Job drawing, mm, ordinate dimensions from the low corner. One solid piece. Give positions to 0.01 mm unless a question says otherwise; leave off trailing zeros. Loops run counter-clockwise (first coordinate to the right, second up) from the corner with the lowest first, then second, coordinate; pieces in that order, holes last. Notation, with made-up numbers: (5, 29.5) -> (40, 29.5) arc R20 cw to (40, 62.5) -> close; hole circle Ø7 at (11, 17). An arc over 180 degrees is marked (long way). Answer as a JSON object with one key per item and string values. Group by question number.
Q1. Drop a flat-ended pin along its axis: pin 1 (1.5 mm diameter, centred on x = 28.5, z = 57, fed in from -Y). Give the stop position or say it passes through.
Q2. Band-saw the part on C-C, the plane y = 0.2. Write the cut outline in (x, z).
Q3. Wall check: probe 1 along X at (y, z) = (0.2, 35); probe 2 along Z at (x, y) = (64, 0.35). Give the ranges that are in metal, low to high. Write a range as from..to.
Q4. Band-saw the part on A-A, the plane z = 35. Write the cut outline in (x, y).
Q5. Band-saw the part on B-B, the plane z = 7.5. Write the cut outline in (x, y).
Q6. Band-saw the part on D-D, the plane x = 7.5. Write the cut outline in (y, z), plus the area to 3 significant figures.
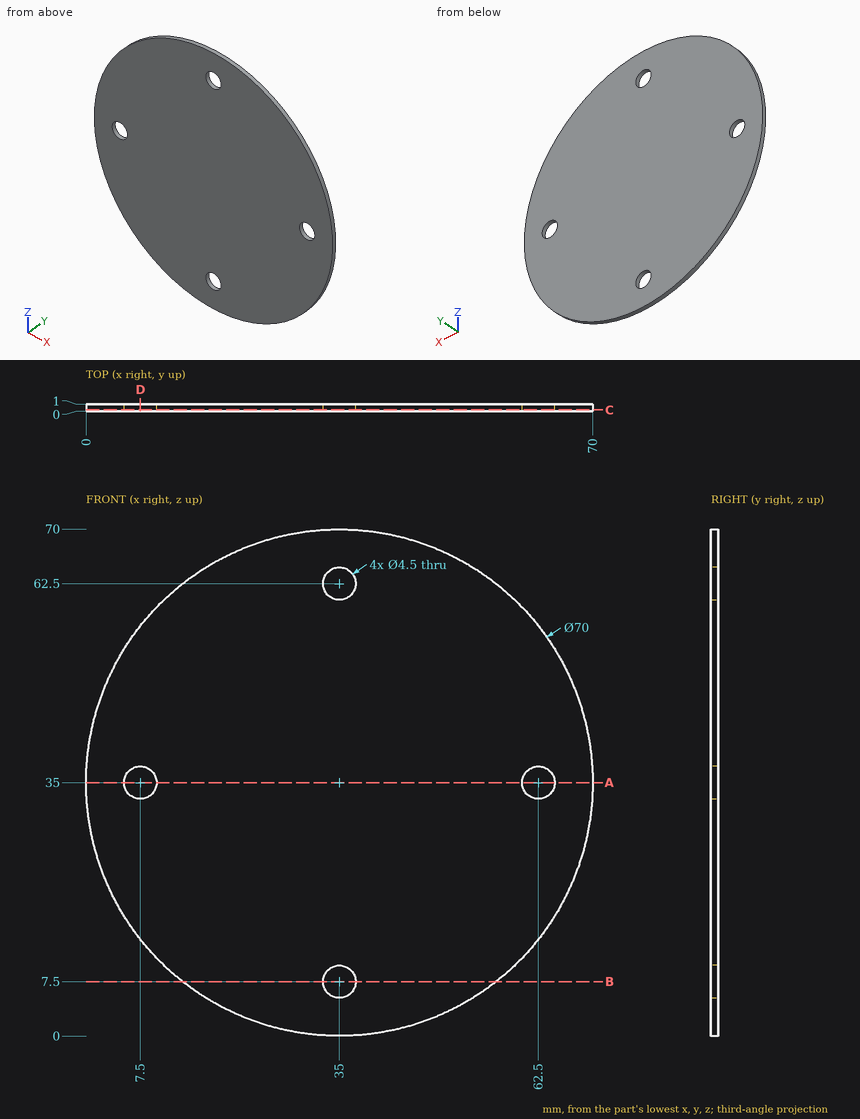
Worked answers:
{
 "1": {"pin 1": "y = 0"},
 "2": {"outline": "circle Ø70 at (35, 35); hole circle Ø4.5 at (7.5, 35); hole circle Ø4.5 at (35, 7.5); hole circle Ø4.5 at (35, 62.5); hole circle Ø4.5 at (62.5, 35)"},
 "3": {"probe 1": "0..5.25, 9.75..60.25, 64.75..70", "probe 2": "15.4..33.32, 36.68..54.6"},
 "4": {"outline": "(0, 0) -> (5.25, 0) -> (5.25, 1) -> (0, 1) -> close; (9.75, 0) -> (60.25, 0) -> (60.25, 1) -> (9.75, 1) -> close; (64.75, 0) -> (70, 0) -> (70, 1) -> (64.75, 1) -> close"},
 "5": {"outline": "(13.35, 0) -> (32.75, 0) -> (32.75, 1) -> (13.35, 1) -> close; (37.25, 0) -> (56.65, 0) -> (56.65, 1) -> (37.25, 1) -> close"},
 "6": {"outline": "(0, 13.35) -> (1, 13.35) -> (1, 32.75) -> (0, 32.75) -> close; (0, 37.25) -> (1, 37.25) -> (1, 56.65) -> (0, 56.65) -> close", "area": "38.8 mm2"}
}
